Here's the drawing with two shaded views (mm, measured from the low corner). I have some questions. A direction names the side the tool comes from. Give positions to 0.01 mm unless a question says otherwise; leave off trailing zeros. Loops run counter-clockwise (first coordinate to the right, second up) from the corner with the lowest first, then second, coordinate; pieces in that order, holes last. Notation, with made-up numbers: M -0.5,80 L 47.5,80 A28 cw 47.5,110 Z; hole C 76,78 d8. An arc over 180 degrees is marked long. Put each result on its own line as item: value. Start each with the question number.
1) Imagine slicing it at C-C (x = 8). Write out the boundary of the cut face in (y, z).
2) Please list where these lines run through material, in increasing order: line 1 along Z through (x, y) = (20, 10.75); line 2 along X through (y, z) = (6.5, 0.95); line 3 along Y through (x, z) = (20, 1.1). Write a range as from..to.
3) For the marked faces 1, 2, 3, 4 and 5, which set-ups out of +Z, -Z, +X, -X, +Y, -Y let a thin tool reach every point of the face, with its end or its side?
4) Imagine slicing it at A-A (z = 14). Write out the boundary of the cut face in (x, y).
5) Imagine slicing it at B-B (y = 6.5). Write out the boundary of the cut face in (x, z), then the cut area to 3 significant figures.
6) For P1, Ø0.9, axis at y = 10.5, z = 9, coming from the +X side; P2, Ø1.5, axis at x = 7.5, y = 2.5, coming from the +Z side; P3, Ø1.3, axis at x = 24, y = 4, coming from the +Z side; P4, Ø7, axis at x = 11.5, z = 9.5, coming from the -Y side, each with a flat end and sliding along its axis, tell me the tip position at first contact or that it passes through.
7) Imagine slicing it at D-D (z = 3.5). Write out the boundary of the cut face in (x, y), then the cut area to 3 significant figures.
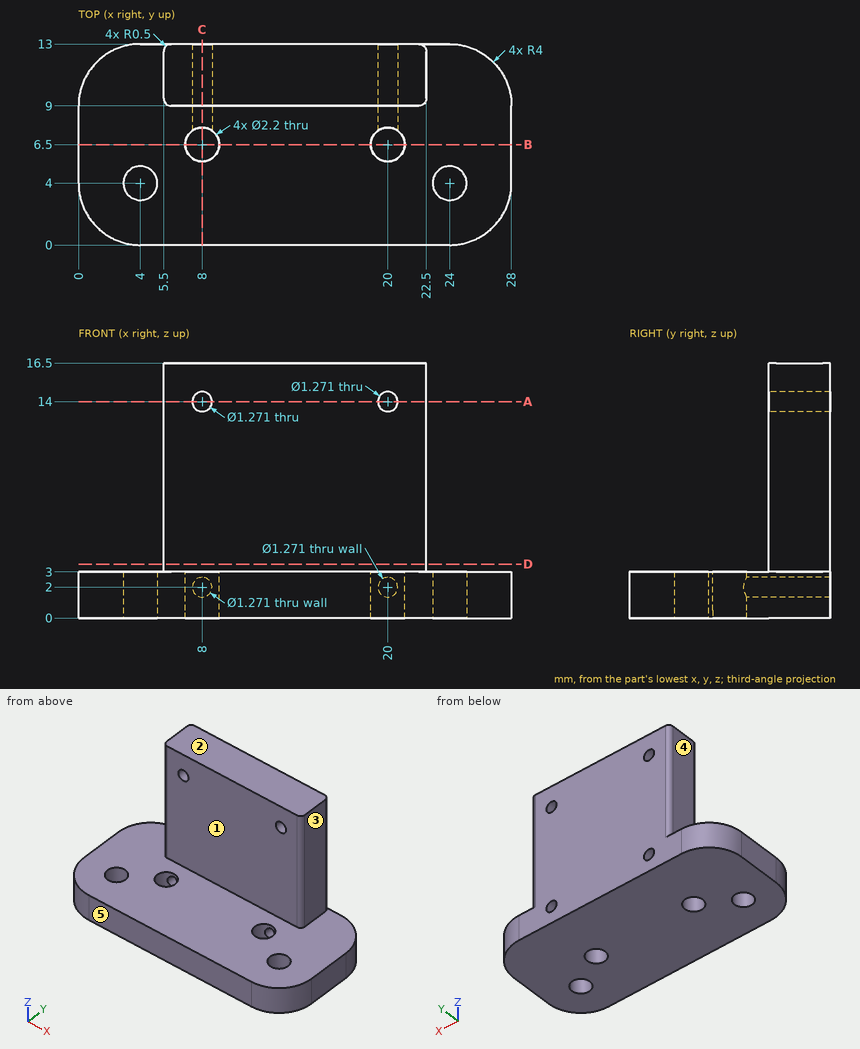
Recorded:
1. outline: M 0,0 L 5.4,0 L 5.4,3 L 0,3 Z; M 7.6,0 L 13,0 L 13,1.36 L 7.6,1.36 Z; M 7.6,2.64 L 13,2.64 L 13,13.36 L 9,13.36 L 9,3 L 7.6,3 Z; M 9,14.64 L 13,14.64 L 13,16.5 L 9,16.5 Z
2. line 1: 0..1.36, 2.64..13.36, 14.64..16.5
2. line 2: 0..6.9, 9.1..18.9, 21.1..28
2. line 3: 0..5.4, 7.6..13
3. face 1: +Z, +X, -X, -Y
3. face 2: +Z, +X, -X, +Y, -Y
3. face 3: +Z, +X, +Y, -Y
3. face 4: +Z, -X, +Y, -Y
3. face 5: +Z, -Z, +X, -X, -Y
4. outline: M 5.5,9.5 A0.5 ccw 6,9 L 7.36,9 L 7.36,13 L 6,13 A0.5 ccw 5.5,12.5 Z; M 8.64,9 L 19.36,9 L 19.36,13 L 8.64,13 Z; M 20.64,9 L 22,9 A0.5 ccw 22.5,9.5 L 22.5,12.5 A0.5 ccw 22,13 L 20.64,13 Z
5. outline: M 0,0 L 6.9,0 L 6.9,3 L 0,3 Z; M 9.1,0 L 18.9,0 L 18.9,3 L 9.1,3 Z; M 21.1,0 L 28,0 L 28,3 L 21.1,3 Z
5. area: 70.8 mm²
6. P1: x = 22.5
6. P2: z = 3
6. P3: through
6. P4: y = 9
7. outline: M 5.5,9.5 A0.5 ccw 6,9 L 22,9 A0.5 ccw 22.5,9.5 L 22.5,12.5 A0.5 ccw 22,13 L 6,13 A0.5 ccw 5.5,12.5 Z
7. area: 67.8 mm²
